Model file for the job. Use its own axes, mm. Face numbers are marked on the shaded views. A direction names the side the tool comes from. Give positions to 0.01 mm unless a question says otherwise; leave off trailing zeros. Write each loop counter-clockwise with the first axis right and the second up, starting at its lowest first coordinate (ties: lowest second). Pieces come first, ordered by that corner, then holes. Notation, with made-up numbers: (-33.5, 65) - (18.5, 65) arc R31 cw to (18.5, 90) - close; hole circle Ø1 at (44, 69). An arc over 180 degrees is marked (long way). Use CSV: the item, a comma, the result in double quotes.
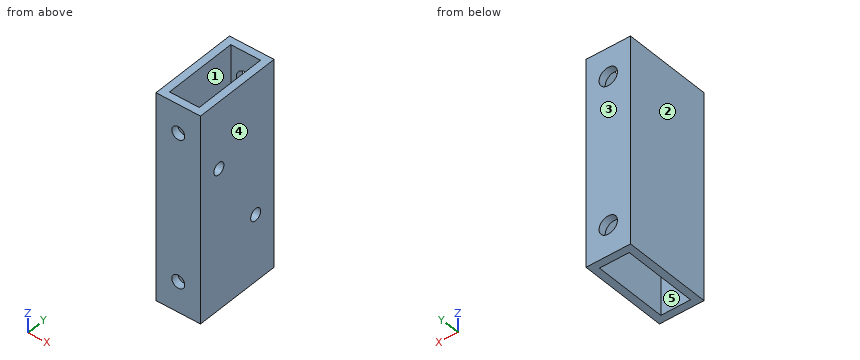
from build123d import *

# Parameters (mm, degrees)
SKETCH1_W           = 19.05
SKETCH1_H           = 38.1
SKETCH1_W_2         = 12.7
SKETCH1_H_2         = 31.75
BOSS_EXTRUDE1_DEPTH = 88.9
SKETCH2_R           = 2.778125
CUT_EXTRUDE1_DEPTH  = 98.188196943
CUT_EXTRUDE2_REACH  = 99.188
SKETCH3_R           = 3.937
CUT_EXTRUDE3_REACH  = 94.892
SKETCH4_R           = 2.5796875


with BuildPart() as part:
    # Sketch1 → Boss-Extrude1 (new body)
    with BuildSketch(Plane.XY):
        Rectangle(SKETCH1_W, SKETCH1_H)
        Rectangle(SKETCH1_W_2, SKETCH1_H_2, mode=Mode.SUBTRACT)
    extrude(amount=BOSS_EXTRUDE1_DEPTH)

    # Sketch2 → Cut-Extrude1 (cut, through all)
    with BuildSketch(Plane(origin=(0, 19.05, 0), x_dir=(1, 0, 0), z_dir=(0, 1, 0))):
        with Locations(Location((0, -76.596875, 0), (0, 0, 270))):
            Circle(SKETCH2_R)
        with Locations(Location((0, -13.096875, 0), (0, 0, 270))):
            Circle(SKETCH2_R)
    extrude(amount=-CUT_EXTRUDE1_DEPTH, mode=Mode.SUBTRACT)

    # Sketch3 → Cut-Extrude2 (cut, up to next)
    with BuildSketch(Plane(origin=(0, 19.05, 0), x_dir=(1, 0, 0), z_dir=(0, 1, 0)), mode=Mode.PRIVATE) as cut_extrude2_sk1:
        with Locations(Location((0, -76.596875, 0), (0, 0, 270))):
            Circle(SKETCH3_R)
    cut_extrude2_tool1 = extrude(cut_extrude2_sk1.sketch, amount=-CUT_EXTRUDE2_REACH, mode=Mode.PRIVATE) & part.part
    # Sketch3 → Cut-Extrude2 (cut, up to next)
    with BuildSketch(Plane(origin=(0, 19.05, 0), x_dir=(1, 0, 0), z_dir=(0, 1, 0)), mode=Mode.PRIVATE) as cut_extrude2_sk2:
        with Locations(Location((0, -13.096875, 0), (0, 0, 270))):
            Circle(SKETCH3_R)
    cut_extrude2_tool2 = extrude(cut_extrude2_sk2.sketch, amount=-CUT_EXTRUDE2_REACH, mode=Mode.PRIVATE) & part.part
    add(cut_extrude2_tool1.solids().sort_by_distance((0, 19.05, 76.596875))[0], mode=Mode.SUBTRACT)
    add(cut_extrude2_tool2.solids().sort_by_distance((0, 19.05, 13.096875))[0], mode=Mode.SUBTRACT)

    # Sketch4 → Cut-Extrude3 (cut, up to next)
    with BuildSketch(Plane(origin=(9.525, 0, 0), x_dir=(0, 0, -1), z_dir=(1, 0, 0)), mode=Mode.PRIVATE) as cut_extrude3_sk1:
        with Locations((-60.325, -9.525)):
            Circle(SKETCH4_R)
    cut_extrude3_tool1 = extrude(cut_extrude3_sk1.sketch, amount=-CUT_EXTRUDE3_REACH, mode=Mode.PRIVATE) & part.part
    # Sketch4 → Cut-Extrude3 (cut, up to next)
    with BuildSketch(Plane(origin=(9.525, 0, 0), x_dir=(0, 0, -1), z_dir=(1, 0, 0)), mode=Mode.PRIVATE) as cut_extrude3_sk2:
        with Locations((-28.575, 9.525)):
            Circle(SKETCH4_R)
    cut_extrude3_tool2 = extrude(cut_extrude3_sk2.sketch, amount=-CUT_EXTRUDE3_REACH, mode=Mode.PRIVATE) & part.part
    add(cut_extrude3_tool1.solids().sort_by_distance((9.525, -9.525, 60.325))[0], mode=Mode.SUBTRACT)
    add(cut_extrude3_tool2.solids().sort_by_distance((9.525, 9.525, 28.575))[0], mode=Mode.SUBTRACT)


solid = part.part
(1) Saw through at B-B, the plane x = 0. List the corners of the cut face in (y, z) (3 decimals).
Checked values:
outline,"(-19.05, 0) - (-15.875, 0) - (-15.875, 10.319) - (-19.05, 10.319) - close; (-19.05, 15.875) - (-15.875, 15.875) - (-15.875, 73.819) - (-19.05, 73.819) - close; (-19.05, 79.375) - (-15.875, 79.375) - (-15.875, 88.9) - (-19.05, 88.9) - close; (15.875, 0) - (19.05, 0) - (19.05, 9.16) - (15.875, 9.16) - close; (15.875, 17.034) - (19.05, 17.034) - (19.05, 72.66) - (15.875, 72.66) - close; (15.875, 80.534) - (19.05, 80.534) - (19.05, 88.9) - (15.875, 88.9) - close"
(2) Saw through at D-D, the plane x = -5.5. List the corners of the cut face in (y, z) (3 decimals), then the cut area to 3 significant figures.
Checked values:
outline,"(-19.05, 0) - (-15.875, 0) - (-15.875, 88.9) - (-19.05, 88.9) - close; (15.875, 0) - (19.05, 0) - (19.05, 88.9) - (15.875, 88.9) - close"
area,"565 mm^2"
(3) Pull direction X, two halves, no side cores. Call the marked faces 3, 4 and 5: released by +X, released by -X, zero draft, split by the parting line, or undercut.
Checked values:
face 3,"zero draft"
face 4,"released by +X"
face 5,"undercut"
(4) 3-axis set-ups, long thin cutter, end or side, ignore diameter. For the marked faces 1 and 2: which of +Z, -Z, +X, -X, +Y, -Y reach the whole face in a straight line?
Checked values:
face 1,"+Z, -Z"
face 2,"+Z, -Z, -X, +Y, -Y"
(5) Saw through at C-C, the plane y = -13. List the corners of the cut face in (x, z) (3 decimals), then the cut area to 3 significant figures.
Checked values:
outline,"(-9.525, 0) - (-6.35, 0) - (-6.35, 88.9) - (-9.525, 88.9) - close; (6.35, 0) - (9.525, 0) - (9.525, 88.9) - (6.35, 88.9) - close"
area,"565 mm^2"
(6) Wall check: probe 1 along X at (y, z) = (-8, 53.5) (3 decimals); probe 2 along Y at (x, z) = (4.5, 24.5) (3 decimals); probe 3 along Y at (x, z) = (2.25, 73.5) (3 decimals). Give the ranges that are in metal, low to high. Write a range as [from, to].
Checked values:
probe 1,"x = [-9.525, -6.35], [6.35, 9.525]"
probe 2,"y = [-19.05, -15.875], [15.875, 19.05]"
probe 3,"y = [-19.05, -15.875]"
(7) Flat gauge pins, fed straight in: P1, Ø6, axis at x = -2.5, y = 2.5, coming from the +Z side; P2, Ø4.5, axis at y = 9.525, z = 28.575, coming from the +X side; P3, Ø7, axis at x = 0, z = 76.6, coming from the +Y side (3 decimals). Where does each tip first touch, or does it go through?
Checked values:
P1,"passes through"
P2,"stops at x = -6.35"
P3,"stops at y = -15.875"
(8) Saw through at A-A, the plane z = 83.5. List the corners of the cut face in (x, y) (3 decimals), then the cut area to 3 significant figures.
Checked values:
outline,"(-9.525, -19.05) - (9.525, -19.05) - (9.525, 19.05) - (-9.525, 19.05) - close; hole (-6.35, -15.875) - (6.35, -15.875) - (6.35, 15.875) - (-6.35, 15.875) - close"
area,"323 mm^2"
